```python
from build123d import *

# Parameters (mm, degrees)
SKETCH1_R           = 65
SKETCH1_R_2         = 60
BOSS_EXTRUDE1_DEPTH = 50
SKETCH2_R           = 65
BOSS_EXTRUDE2_DEPTH = 20
SKETCH3_R           = 4.1
SKETCH3_W           = 45
SKETCH3_H           = 45
CUT_EXTRUDE1_DEPTH  = 116.542200083
SKETCH5_W           = 45
SKETCH5_H           = 25
CUT_EXTRUDE2_DEPTH  = 15
SKETCH6_R           = 50
CUT_EXTRUDE3_DEPTH  = 6
SKETCH7_R           = 7
SKETCH7_R_2         = 4.1
BOSS_EXTRUDE3_DEPTH = 6
SKETCH8_R           = 39
CUT_EXTRUDE4_DEPTH  = 10


with BuildPart() as part:
    # Sketch1 → Boss-Extrude1 (new body)
    with BuildSketch(Plane(origin=(0, 0, 0), x_dir=(1, 0, 0), z_dir=(0, 1, 0))):
        with Locations(Location((0, 0, 0), (0, 0, 270))):
            Circle(SKETCH1_R)
        with Locations(Location((0, 0, 0), (0, 0, 270))):
            Circle(SKETCH1_R_2, mode=Mode.SUBTRACT)
    extrude(amount=BOSS_EXTRUDE1_DEPTH)

    # Sketch2 → Boss-Extrude2 (add)
    with BuildSketch(Plane(origin=(0, 50, 0), x_dir=(1, 0, 0), z_dir=(0, 1, 0))):
        with Locations(Location((0, 0, 0), (0, 0, 270))):
            Circle(SKETCH2_R)
    extrude(amount=BOSS_EXTRUDE2_DEPTH)

    # Sketch3 → Cut-Extrude1 (cut, through all)
    with BuildSketch(Plane(origin=(0, 70, 0), x_dir=(1, 0, 0), z_dir=(0, 1, 0))):
        with Locations(Location((-33.234018716, -33.234018716, 0), (0, 0, 270))):
            Circle(SKETCH3_R)
        with Locations(Location((-33.234018716, 33.234018716, 0), (0, 0, 270))):
            Circle(SKETCH3_R)
        with Locations(Location((33.234018716, 33.234018716, 0), (0, 0, 270))):
            Circle(SKETCH3_R)
        with Locations(Location((33.234018716, -33.234018716, 0), (0, 0, 270))):
            Circle(SKETCH3_R)
        Rectangle(SKETCH3_W, SKETCH3_H)
    extrude(amount=-CUT_EXTRUDE1_DEPTH, mode=Mode.SUBTRACT)

    # Sketch5 → Cut-Extrude2 (cut)
    with BuildSketch(Plane.XZ.offset(-50)):
        with Locations((0, 35)):
            Rectangle(SKETCH5_W, SKETCH5_H)
    extrude(amount=-CUT_EXTRUDE2_DEPTH, mode=Mode.SUBTRACT)

    # Sketch6 → Cut-Extrude3 (cut)
    with BuildSketch(Plane.XZ.offset(-50)):
        Circle(SKETCH6_R)
    extrude(amount=-CUT_EXTRUDE3_DEPTH, mode=Mode.SUBTRACT)

    # Sketch7 → Boss-Extrude3 (add)
    # profile 1 of 4: a face of its own
    with BuildSketch(Plane.XZ.offset(-56)):
        with Locations((-33.234018716, -33.234018716)):
            Circle(SKETCH7_R)
        with Locations(Location((-33.234018716, -33.234018716, 0), (0, 0, 90))):
            Circle(SKETCH7_R_2, mode=Mode.SUBTRACT)
    # profile 2 of 4: a face of its own
    with BuildSketch(Plane.XZ.offset(-56)):
        with Locations((-33.234018716, 33.234018716)):
            Circle(SKETCH7_R)
        with Locations(Location((-33.234018716, 33.234018716, 0), (0, 0, 90))):
            Circle(SKETCH7_R_2, mode=Mode.SUBTRACT)
    # profile 3 of 4: a face of its own
    with BuildSketch(Plane.XZ.offset(-56)):
        with Locations((33.234018716, -33.234018716)):
            Circle(SKETCH7_R)
        with Locations(Location((33.234018716, -33.234018716, 0), (0, 0, 90))):
            Circle(SKETCH7_R_2, mode=Mode.SUBTRACT)
    # profile 4 of 4: a face of its own
    with BuildSketch(Plane.XZ.offset(-56)):
        with Locations((33.234018716, 33.234018716)):
            Circle(SKETCH7_R)
        with Locations(Location((33.234018716, 33.234018716, 0), (0, 0, 90))):
            Circle(SKETCH7_R_2, mode=Mode.SUBTRACT)
    extrude(amount=BOSS_EXTRUDE3_DEPTH)

    # Sketch8 → Cut-Extrude4 (cut)
    with BuildSketch(Plane.XZ.offset(-56)):
        with Locations(Location((0, 0, 0), (0, 0, 270))):
            Circle(SKETCH8_R)
    extrude(amount=-CUT_EXTRUDE4_DEPTH, mode=Mode.SUBTRACT)


solid = part.part
```
Here's how the part is built. I have some questions about the finished solid (model axes, mm). A direction names the side the tool comes from. Coordinates: 2 decimals unless noted, no trailing zeros. Order: outer loops, then holes, each group sorted by start corner. A loop starts at its lowest first (then second) coordinate and runs counter-clockwise, first axis right, second up.
1) Imagine slicing it at C-C on y = 30. List the corners of the cut face in (x, z) for me, and give its area (3 significant figures).
2) Imagine slicing it at D-D on x = 53. List the corners of the cut face in (y, z) for me.
3) Imagine slicing it at A-A on x = 0. List the corners of the cut face in (y, z) for me.
4) I need wall thicknesses on line 1 (X direction, y = 30, z = 0); line 2 (Y direction, x = 13, z = 54); line 3 (Y direction, x = -27.5, z = -14). Which ranges of each line are inside material? Lowest first, please.
5) Imagine slicing it at B-B on z = 0. List the corners of the cut face in (x, y) for me.
6) Will these pins go through, and if not, where does the flat tip stop? pin 1 (8 mm diameter, centred on y = 56, z = 46, fed in from +X); pin 2 (6 mm diameter, centred on y = 36.5, z = 2, fed in from -X); pin 3 (8 mm diameter, centred on x = -0.5, z = 39.5, fed in from -Y); pin 4 (13 mm diameter, centred on x = -33.23, z = -33.23, fed in from +Y).
7) Which directions (+Z, -Z, +X, -X, +Y, -Y) give clear straight access to the entire face, cutting with the end or side of a thin tool? Please do faces 1 (the face through (-25, 66, 1)), 2 (the face through (1, 70, 28)), 3 (the face through (0, 68, -22.5)).
Response values:
1. outline: circle Ø130 at (0, 0); hole circle Ø120 at (0, 0)
1. area: 1,960 mm2
2. outline: (0, -37.63) - (70, -37.63) - (70, 37.63) - (0, 37.63) - (0, 28.12) - (50, 28.12) - (50, -28.12) - (0, -28.12) - close
3. outline: (0, -65) - (70, -65) - (70, -22.5) - (66, -22.5) - (66, -39) - (56, -39) - (56, -50) - (50, -50) - (50, -60) - (0, -60) - close; (0, 60) - (50, 60) - (50, 50) - (56, 50) - (56, 47.5) - (65, 47.5) - (65, 39) - (66, 39) - (66, 22.5) - (70, 22.5) - (70, 65) - (0, 65) - close
4. line 1: x = -65 to -60, 60 to 65
4. line 2: y = 50 to 70
4. line 3: y = 66 to 70
5. outline: (-65, 0) - (-60, 0) - (-60, 50) - (-50, 50) - (-50, 56) - (-39, 56) - (-39, 66) - (-22.5, 66) - (-22.5, 70) - (-65, 70) - close; (22.5, 66) - (39, 66) - (39, 56) - (50, 56) - (50, 50) - (60, 50) - (60, 0) - (65, 0) - (65, 70) - (22.5, 70) - close
6. pin 1: stops at x = 49.61
6. pin 2: stops at x = -65
6. pin 3: stops at y = 65
6. pin 4: stops at y = 70
7. face 1: -Y
7. face 2: +Z, -Z, +X, -X, +Y
7. face 3: +Y, -Y
